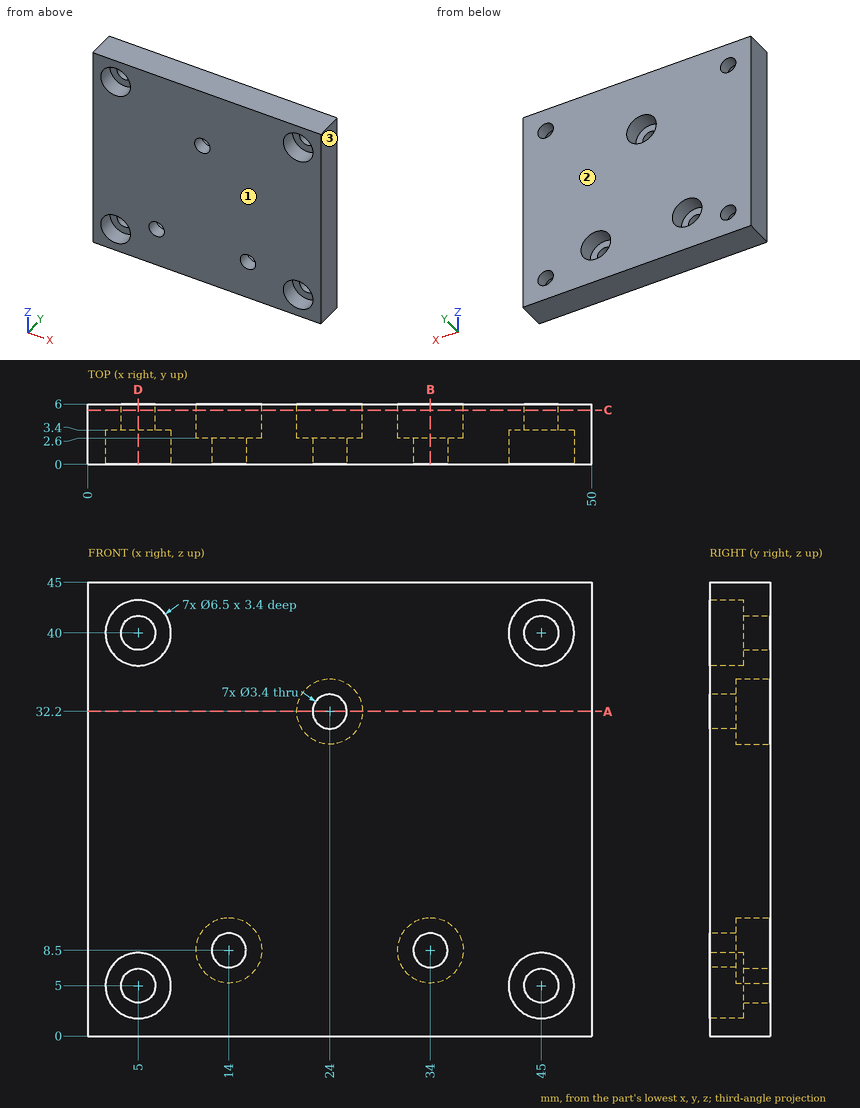
Design review of the part shown in the three views and the two pictorial views. Dimensions are in mm from the part's minimum x, y and z. Round coordinates to 2 decimals unless told otherwise and drop trailing zeros. Loops run counter-clockwise (first coordinate to the right, second up) from the corner with the lowest first, then second, coordinate; pieces in that order, holes last. Notation, with made-up numbers: (26.25, 48) -> (40.25, 48) arc R24 cw to (40.25, 80) -> close; hole circle Ø11 at (49, 83). An arc over 180 degrees is marked (long way). Use one line per item in the form item = value. Start each with the question number.
Q1. For pin 1 Ø3 at (x, z) = (45, 40) entering from -Y; pin 2 Ø5.5 at (x, z) = (24, 32.2) entering from +Y; pin 3 Ø2 at (x, z) = (4, 5.5) entering from -Y, all flat-tipped, find the tip position at first contact; note any pin that passes through.
Q2. We need section B-B on x = 34. Give the boundary of the cut face in (y, z).
Q3. Wall thickness on line 1 along X through (y, z) = (0.85, 8.5); line 2 along X through (y, z) = (2.05, 5); line 3 along X through (y, z) = (2.8, 30.5): over which ranges is each line inside the solid? List them lowest first. Write a range as [from, to].
Q4. We need section D-D on x = 5. Give the boundary of the cut face in (y, z).
Q5. Draft analysis for pull direction Y (two halves, no side actions). For the marked faces 1, 2 and 3, state which applies: +Y half, -Y half, draft (parallel to the pull), parting line (faces both ways), or undercut.
Q6. We need section A-A on z = 32.2. Give the boundary of the cut face in (x, y).
Q7. We need section C-C on y = 5.4. Give the boundary of the cut face in (x, z).
Calculated:
q1.pin_1 = through
q1.pin_2 = 2.6
q1.pin_3 = 3.4
q2.outline = (0, 0) -> (6, 0) -> (6, 5.25) -> (2.6, 5.25) -> (2.6, 6.8) -> (0, 6.8) -> close; (0, 10.2) -> (2.6, 10.2) -> (2.6, 11.75) -> (6, 11.75) -> (6, 45) -> (0, 45) -> close
q3.line_1 = [0, 12.3], [15.7, 32.3], [35.7, 50]
q3.line_2 = [0, 1.75], [8.25, 41.75], [48.25, 50]
q3.line_3 = [0, 21.23], [26.77, 50]
q4.outline = (0, 0) -> (6, 0) -> (6, 3.3) -> (3.4, 3.3) -> (3.4, 1.75) -> (0, 1.75) -> close; (0, 8.25) -> (3.4, 8.25) -> (3.4, 6.7) -> (6, 6.7) -> (6, 38.3) -> (3.4, 38.3) -> (3.4, 36.75) -> (0, 36.75) -> close; (0, 43.25) -> (3.4, 43.25) -> (3.4, 41.7) -> (6, 41.7) -> (6, 45) -> (0, 45) -> close
q5.face_1 = -Y half
q5.face_2 = +Y half
q5.face_3 = draft
q6.outline = (0, 0) -> (22.3, 0) -> (22.3, 2.6) -> (20.75, 2.6) -> (20.75, 6) -> (0, 6) -> close; (25.7, 0) -> (50, 0) -> (50, 6) -> (27.25, 6) -> (27.25, 2.6) -> (25.7, 2.6) -> close
q7.outline = (0, 0) -> (50, 0) -> (50, 45) -> (0, 45) -> close; hole circle Ø3.4 at (5, 5); hole circle Ø3.4 at (5, 40); hole circle Ø6.5 at (14, 8.5); hole circle Ø6.5 at (24, 32.2); hole circle Ø6.5 at (34, 8.5); hole circle Ø3.4 at (45, 5); hole circle Ø3.4 at (45, 40)
